Can you work these out from the drawing? Everything is in mm from the part's minimum corner. A direction names the side the tool comes from. Round coordinates to 2 decimals unless told otherwise and drop trailing zeros. Write each loop counter-clockwise with the first axis right and the second up, starting at its lowest first coordinate (ties: lowest second). Pieces come first, ordered by that corner, then holes. Notation, with made-up numbers: (53, 88) -> (92, 88) arc R26 cw to (92, 109) -> close; hole circle Ø7 at (-8.75, 81). An arc over 180 degrees is marked (long way). Answer as CSV lines item,"result". Start each with the question number.
Q1. If we mould it in two halves opening along Y, with no side actions, what happens to the marked faces 1, 2 and 3? For each: pulls with the +Y half, pulls with the -Y half, needs draft (parallel to the pull), parting line crosses it, or undercut.
Q2. Imagine slicing it at C-C on z = 4.45. Please give me the cut outline in (x, y).
Q3. Imagine slicing it at B-B on x = 8.25. Please give me the cut outline in (y, z).
Q4. Imagine slicing it at D-D on z = 1.4. Please give me the cut outline in (x, y).
Q5. Imagine slicing it at A-A on y = 2. Please give me the cut outline in (x, z), and give its area (3 significant figures).
Q6. Will these pins go through, and if not, where does the flat tip stop? pin 1 Ø2 at (y, z) = (1.5, 4.5) entering from -X; pin 2 Ø2 at (x, y) = (6, 2.5) entering from +Z.
Q7. If I drill on line 1 (Y direction, x = 9.6, z = 4); line 2 (Z direction, x = 5, y = 6); line 3 (X direction, y = 3.75, z = 4.9), over which ranges is the centre line in solid material (lowest first)? Write a range as [from, to].
Q8. For the marked faces 4 and 5, which set-ups out of +Z, -Z, +X, -X, +Y, -Y let a thin tool reach every point of the face, with its end or its side?
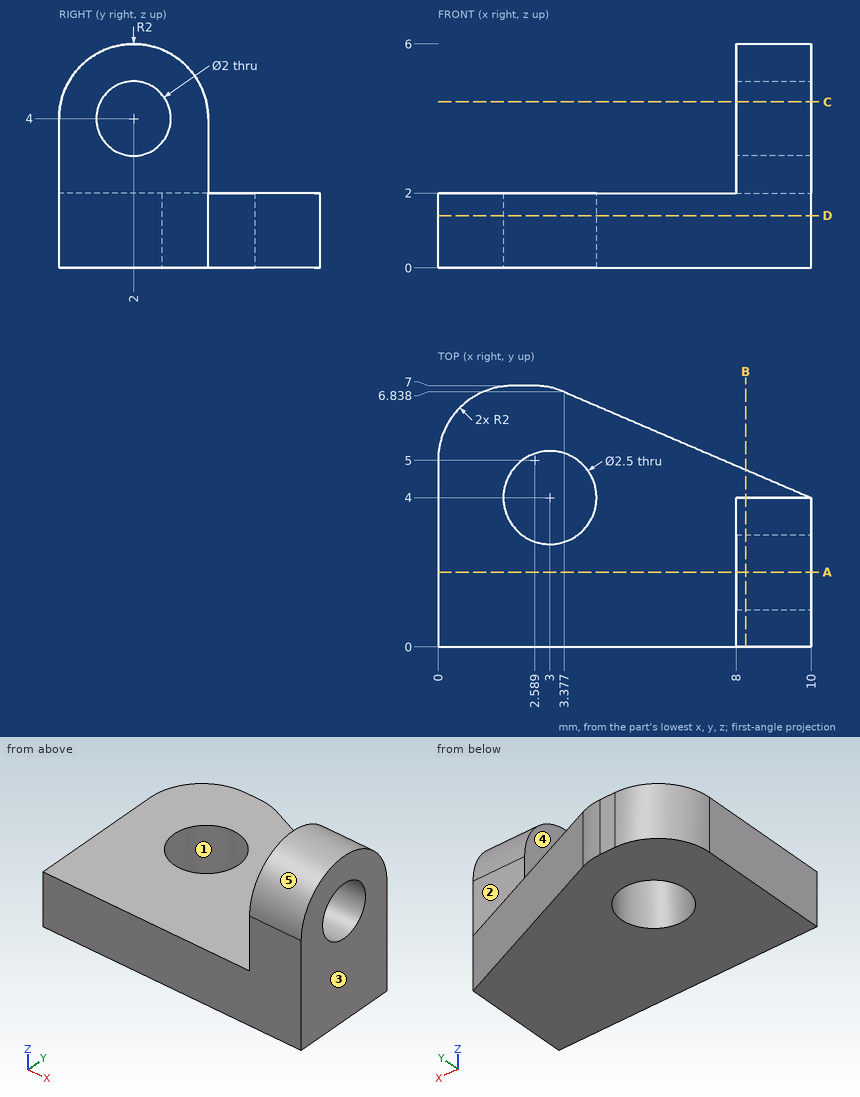
Checks:
1,face 1,"undercut"
1,face 2,"pulls with the +Y half"
1,face 3,"needs draft"
2,outline,"(8, 0.05) -> (10, 0.05) -> (10, 1.11) -> (8, 1.11) -> close; (8, 2.89) -> (10, 2.89) -> (10, 3.95) -> (8, 3.95) -> close"
3,outline,"(0, 0) -> (4.75, 0) -> (4.75, 2) -> (4, 2) -> (4, 4) arc R2 ccw to (0, 4) -> close; hole circle Ø2 at (2, 4)"
4,outline,"(0, 0) -> (10, 0) -> (10, 4) -> (3.38, 6.84) arc R2 ccw to (2.59, 7) -> (2, 7) arc R2 ccw to (0, 5) -> close; hole circle Ø2.5 at (3, 4)"
5,outline,"(0, 0) -> (10, 0) -> (10, 3) -> (8, 3) -> (8, 2) -> (0, 2) -> close; (8, 5) -> (10, 5) -> (10, 6) -> (8, 6) -> close"
5,area,"24.0 mm^2"
6,pin 1,"x = 8"
6,pin 2,"z = 2"
7,line 1,"[0, 1], [3, 4]"
7,line 2,"[0, 2]"
7,line 3,"[8, 10]"
8,face 4,"+Z, -X, +Y, -Y"
8,face 5,"+Z, +X, -X"
